Input: part model. Units: mm. Frame: model coordinates. Face numbers are marked on the shaded views. A direction names the side the tool comes from. Give positions to 0.01 mm unless a question says otherwise; leave off trailing zeros. Loops run counter-clockwise (first coordinate to the right, second up) from the corner with the lowest first, then second, coordinate; pieces in that order, holes last. Notation, with made-up numbers: (44.25, 87) -> (91.25, 87) arc R27 cw to (91.25, 118) -> close; hole circle Ø4 at (-10.75, 39). An arc over 180 degrees is marked (long way). Answer as a JSON object with one key per item and string values. Group by question number.
```python
from build123d import *

# Parameters (mm, degrees)
CYLINDER001_R     = 1.5
CYLINDER001_DEPTH = 10
CYLINDER002_R     = 1.5
CYLINDER002_DEPTH = 10
BOX_W             = 10
BOX_H             = 42
BOX_DEPTH         = 10


with BuildPart() as zylinder001:
    # Cylinder001 → Cylinder001 (new body)
    with BuildSketch(Plane(origin=(1.5, 42, 0), x_dir=(1, 0, 0), z_dir=(0, 0, 1))):
        Circle(CYLINDER001_R)
    extrude(amount=CYLINDER001_DEPTH)


with BuildPart() as zylinder002:
    # Cylinder002 → Cylinder002 (new body)
    with BuildSketch(Plane(origin=(8.5, 42, 0), x_dir=(1, 0, 0), z_dir=(0, 0, 1))):
        Circle(CYLINDER002_R)
    extrude(amount=CYLINDER002_DEPTH)


with BuildPart() as fusion:
    # Box → Box (new body)
    with BuildSketch(Plane.XY):
        with Locations((5, 21)):
            Rectangle(BOX_W, BOX_H)
    extrude(amount=BOX_DEPTH)

    # Fusion: union Zylinder001, Zylinder002
    add(zylinder001.part)
    add(zylinder002.part)


solid = fusion.part
```
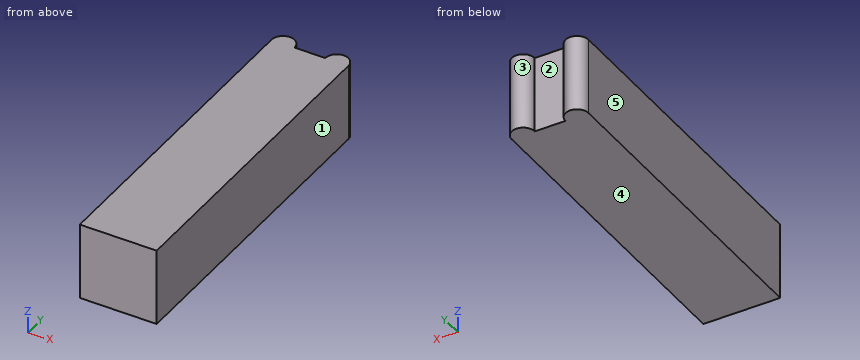
Q1. Ray query, probe 1 along Y at (x, z) = (3.75, 1); probe 2 along Y at (x, z) = (0.75, 6.25). Return the intervals inside material, ascending.
Q2. Section A-A on z = 2.5. Return the cut outline in (x, y), then the cut area to 3 significant figures.
Q3. Pin query (flat end, axial travel): pin 1 Ø3 at (x, z) = (4, 8.5) entering from +Y; pin 2 Ø1.2 at (x, z) = (5, 5.5) entering from +Y; pin 3 Ø1.5 at (x, z) = (7.5, 2) entering from +Y. Return the tip coordinate at first contact, or that it passes through.
Q4. Pull-direction query (X, two-part tool) for the marked faces 3, 4 and 5; classes: +X half, -X half, draft (parallel to the pull), parting line (faces both ways), or undercut.
Q5. Section B-B on x = 4. Return the cut outline in (y, z), then the cut area to 3 significant figures.
Q6. Set-up query: the marked faces 1 and 2. Return all of +Z, -Z, +X, -X, +Y, -Y with unobstructed straight access to the full face (end or side cutting, diameter ignored); none if empty.
Numbers:
{
 "1": {"probe 1": "y = 0 to 42", "probe 2": "y = 0 to 43.3"},
 "2": {"outline": "(0, 0) -> (10, 0) -> (10, 42) arc R1.5 ccw to (7, 42) -> (3, 42) arc R1.5 ccw to (0, 42) -> close", "area": "427 mm²"},
 "3": {"pin 1": "stops at y = 43.12", "pin 2": "stops at y = 42", "pin 3": "stops at y = 43.48"},
 "4": {"face 3": "undercut", "face 4": "draft", "face 5": "-X half"},
 "5": {"outline": "(0, 0) -> (42, 0) -> (42, 10) -> (0, 10) -> close", "area": "420 mm²"},
 "6": {"face 1": "+Z, -Z, +X, +Y, -Y", "face 2": "+Z, -Z, +Y"}
}
